from build123d import *

# Parameters (mm, degrees)
BOSS_EXTRUDE1_DEPTH      = 3.571875
BOSS_EXTRUDE1_DEPTH_BACK = 0.254
SKETCH1_R                = 4.7625
SKETCH2_R                = 3.96875
BOSS_EXTRUDE2_DEPTH      = 13.890625
SKETCH3_R                = 2.38125
CUT_EXTRUDE1_DEPTH       = 19.953553354
CHAMFER1_SIZE            = 0.127


with BuildPart() as part:
    # Sketch1 → Boss-Extrude1 (new, two sides: drawn at the far end of the back side and taken through both)
    with BuildSketch(Plane(origin=(0, 0, 0), x_dir=(1, 0, 0), z_dir=(0, 1, 0)).offset(-BOSS_EXTRUDE1_DEPTH_BACK)):
        with Locations(Location((0, 0, 0), (0, 0, 270))):
            Circle(SKETCH1_R)
    extrude(amount=BOSS_EXTRUDE1_DEPTH + BOSS_EXTRUDE1_DEPTH_BACK)

    # Sketch2 → Boss-Extrude2 (add)
    with BuildSketch(Plane.XZ.offset(0.254)):
        with Locations(Location((0, 0, 0), (0, 0, 270))):
            Circle(SKETCH2_R)
    extrude(amount=BOSS_EXTRUDE2_DEPTH)

    # Sketch3 → Cut-Extrude1 (cut, through all)
    with BuildSketch(Plane.XZ.offset(14.144625)):
        with Locations(Location((0, 0, 0), (0, 0, 270))):
            Circle(SKETCH3_R)
    extrude(amount=-CUT_EXTRUDE1_DEPTH, mode=Mode.SUBTRACT)

    # Chamfer1
    chamfer1_edges = [part.edges().sort_by_distance(p)[0] for p in [
        (0, -14.144625, 3.96875),
    ]]
    chamfer(chamfer1_edges, length=CHAMFER1_SIZE)


solid = part.part
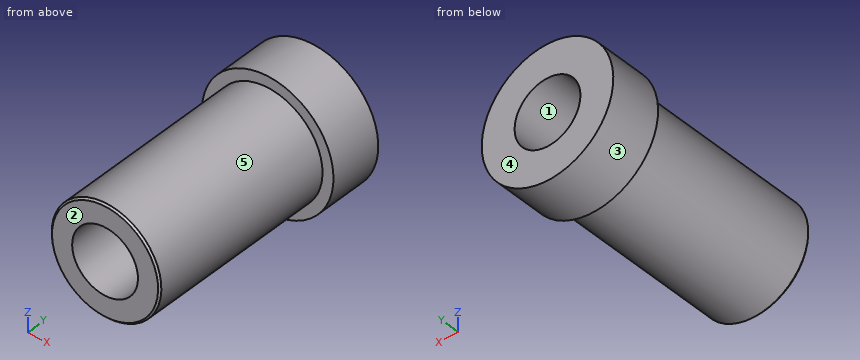
Input: part model. Units: mm. Frame: model coordinates. Face numbers are marked on the shaded views. A direction names the side the tool comes from. Round coordinates to 2 decimals unless told otherwise and drop trailing zeros. Loops run counter-clockwise (first coordinate to the right, second up) from the corner with the lowest first, then second, coordinate; pieces in that order, holes last. Notation, with made-up numbers: M -40,85.5 L -31,85.5 A26 cw -31,117.5 Z; hole C 62.5,86 d7. An arc over 180 degrees is marked long. Answer as CSV lines item,"result". Start each with the question number.
(1) First-contact query: pin 1 (4 mm diameter, centred on y = -11, z = -1.5, fed in from -X); pin 2 (1 mm diameter, centred on y = -9, z = -3.5, fed in from +X). Flat tips, straight axial feed; report the tip coordinate or a pass-through.
(2) Section A-A, the plane x = 0. Output: boundary loops of the cut face in (y, z).
(3) Line query: line 1 (X direction, y = -5.25, z = 0); line 2 (X direction, y = -6.5, z = -0.5). Output: solid intervals per line, ascending. Write a range as [from, to].
(4) Section B-B, the plane z = 0. Output: boundary loops of the cut face in (x, y), plus the area to 3 significant figures.
(5) Reachability of the marked faces 4 and 5 from +Z, -Z, +X, -X, +Y, -Y: full face, straight path, thin tool, end or side. Return the list, or none.
(6) Draft query along X for the marked faces 1, 2 and 3. Return one class per face: released by +X, released by -X, zero draft, split by the parting line, or undercut.
(7) Section C-C, the plane y = -11.5. Output: boundary loops of the cut face in (x, z), plus the area to 3 significant figures.
Values found:
1,pin 1,"stops at x = -3.97"
1,pin 2,"stops at x = 2.6"
2,outline,"M -14.14,-3.84 L -14.02,-3.97 L -0.25,-3.97 L -0.25,-4.76 L 3.57,-4.76 L 3.57,-2.38 L -14.14,-2.38 Z; M -14.14,2.38 L 3.57,2.38 L 3.57,4.76 L -0.25,4.76 L -0.25,3.97 L -14.02,3.97 L -14.14,3.84 Z"
3,line 1,"x = [-3.97, -2.38], [2.38, 3.97]"
3,line 2,"x = [-3.94, -2.33], [2.33, 3.94]"
4,outline,"M -4.76,-0.25 L -3.97,-0.25 L -3.97,-14.02 L -3.84,-14.14 L -2.38,-14.14 L -2.38,3.57 L -4.76,3.57 Z; M 2.38,-14.14 L 3.84,-14.14 L 3.97,-14.02 L 3.97,-0.25 L 4.76,-0.25 L 4.76,3.57 L 2.38,3.57 Z"
4,area,"62.3 mm²"
5,face 4,"+Z, -Z, +X, -X, +Y"
5,face 5,"-Y"
6,face 1,"undercut"
6,face 2,"zero draft"
6,face 3,"split by the parting line"
7,outline,"C 0,0 d7.94; hole C 0,0 d4.76"
7,area,"31.7 mm²"
